Here's the drawing with two shaded views (mm, measured from the low corner). I have some questions. A direction names the side the tool comes from. Coordinates: 2 decimals unless noted, no trailing zeros. Write each loop counter-clockwise with the first axis right and the second up, starting at its lowest first coordinate (ties: lowest second). Pieces come first, ordered by that corner, then holes. Notation, with made-up numbers: (-22, 18.5) -> (-1, 18.5) arc R16 ccw to (-1, 32.5) -> close; hole circle Ø10 at (74, 58). An arc over 180 degrees is marked (long way). Use one line per item in the form item = value.
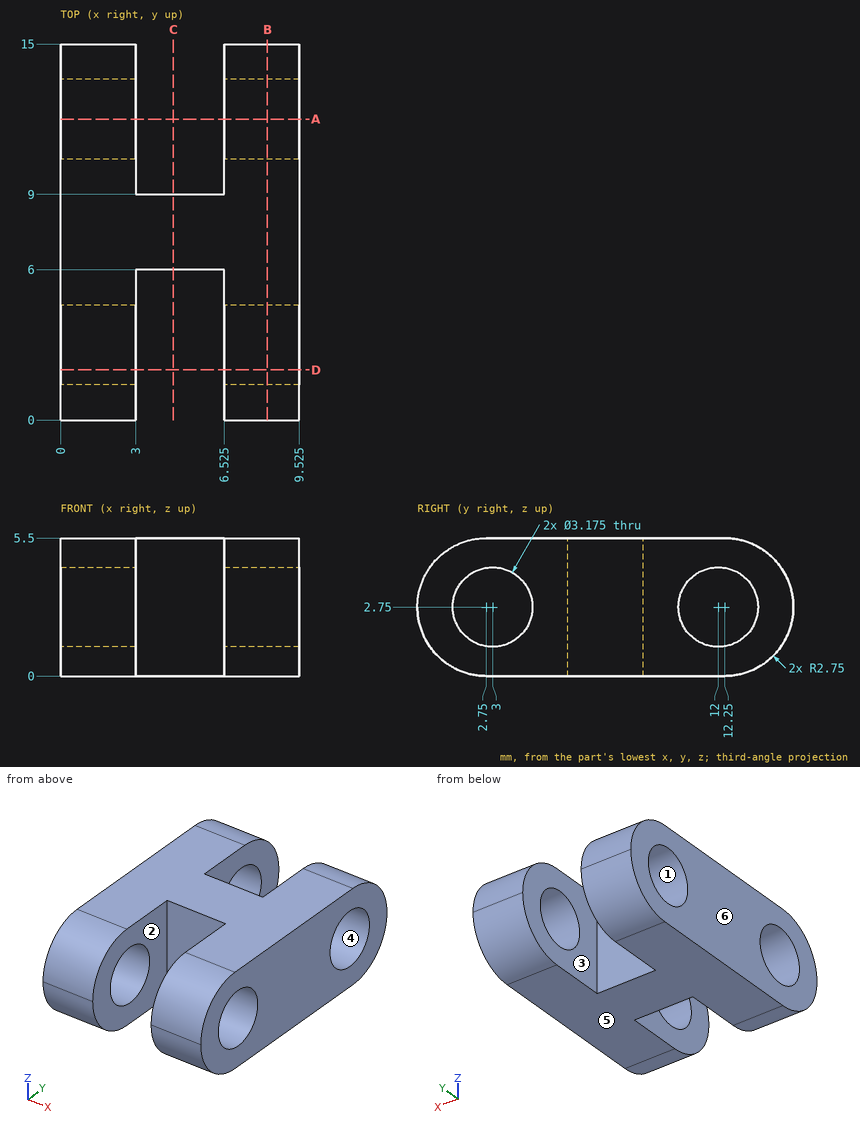
Q1. Suppose I cut it at C-C (x = 4.5). Write out the boundary of the cut face in (y, z), then the cut area to 3 significant figures.
Return value:
outline = (6, 0) -> (9, 0) -> (9, 5.5) -> (6, 5.5) -> close
area = 16.5 mm2
Q2. For the marked faces 1, 2 and 3, which set-ups out of +Z, -Z, +X, -X, +Y, -Y let a thin tool reach every point of the face, with its end or its side?
Return value:
face_1 = +X, -X
face_2 = +Z, -Z, -Y
face_3 = +Z, -Z, +Y
Q3. Suppose I cut it at A-A (y = 12). Write out the boundary of the cut face in (x, z) (1 decimal), then the cut area to 4 significant figures.
Return value:
outline = (0, 0) -> (3, 0) -> (3, 1.2) -> (0, 1.2) -> close; (0, 4.3) -> (3, 4.3) -> (3, 5.5) -> (0, 5.5) -> close; (6.5, 0) -> (9.5, 0) -> (9.5, 1.2) -> (6.5, 1.2) -> close; (6.5, 4.3) -> (9.5, 4.3) -> (9.5, 5.5) -> (6.5, 5.5) -> close
area = 13.95 mm2
Q4. Thinking about a two-plate mould opening in Z: for the marked faces 4, 5 and 6, which applies, released by +Z, released by -Z, zero draft, split by the parting line, or undercut?
Return value:
face_4 = undercut
face_5 = released by -Z
face_6 = zero draft
Q5. Suppose I cut it at D-D (y = 2). Write out the boundary of the cut face in (x, z) (3 decimals).
Return value:
outline = (0, 0.104) -> (3, 0.104) -> (3, 1.517) -> (0, 1.517) -> close; (0, 3.983) -> (3, 3.983) -> (3, 5.396) -> (0, 5.396) -> close; (6.525, 0.104) -> (9.525, 0.104) -> (9.525, 1.517) -> (6.525, 1.517) -> close; (6.525, 3.983) -> (9.525, 3.983) -> (9.525, 5.396) -> (6.525, 5.396) -> close
Q6. If I drill on line 1 (Y direction, x = 1, z = 2.75); line 2 (X direction, y = 13.5, z = 1.8) (3 decimals); line 3 (Y direction, x = 3.75, z = 0.8), over which ranges is the centre line in solid material (lowest first)? Write a range as from..to.
Return value:
line_1 = 0..1.41, 4.59..10.41, 13.59..15
line_2 = 0..3, 6.525..9.525
line_3 = 6..9
Q7. Suppose I cut it at B-B (x = 8.25). Give the number of separate pieces and of enclosed holes in the cut face, then the cut area to 3 significant figures.
Return value:
separate_pieces = 1
enclosed_holes = 2
area = 60.2 mm2
Q8. Will this pin go through, and if not, where does the flat tip stop? pin 1 (1 mm diameter, centred on x = 5.5, z = 3, fed in from +Y).
Return value:
pin_1 = 9
